from build123d import *

# Parameters (mm, degrees)
SKETCH1_W               = 70
SKETCH1_H               = 80
BOSS_EXTRUDE1_DEPTH     = 6.8
SKETCH2_W               = 54
SKETCH2_H               = 73
CUT_EXTRUDE1_DEPTH      = 107.518730747
SKETCH3_R               = 2.5
CUT_EXTRUDE2_DEPTH      = 107.518730747
LPATTERN1_COUNT         = 4
LPATTERN1_PITCH         = 16.72
MIRROR1_COPY_1_SKETCH_R = 2.5
MIRROR1_COPY_1_DEPTH    = 107.518730747
MIRROR1_COPY_2_SKETCH_R = 2.5
MIRROR1_COPY_2_DEPTH    = 107.518730747
MIRROR1_COPY_3_SKETCH_R = 2.5
MIRROR1_COPY_3_DEPTH    = 107.518730747
SKETCH5_W               = 8.11
SKETCH5_H               = 73
CUT_EXTRUDE3_DEPTH      = 2.8
SKETCH4_W               = 20
SKETCH4_H               = 8
BOSS_EXTRUDE2_DEPTH     = 6.8
SKETCH7_R               = 2.25
CUT_EXTRUDE4_DEPTH      = 6.8
FILLET1_R               = 1
FILLET2_R               = 1
FILLET3_R               = 5


with BuildPart() as part:
    # Sketch1 → Boss-Extrude1 (new body)
    with BuildSketch(Plane(origin=(0, 0, 0), x_dir=(1, 0, 0), z_dir=(0, 1, 0))):
        with Locations((35, -40)):
            Rectangle(SKETCH1_W, SKETCH1_H)
    extrude(amount=BOSS_EXTRUDE1_DEPTH)

    # Sketch2 → Cut-Extrude1 (cut, through all)
    with BuildSketch(Plane(origin=(0, 6.8, 0), x_dir=(1, 0, 0), z_dir=(0, 1, 0))):
        with Locations((35.11, -43.5)):
            Rectangle(SKETCH2_W, SKETCH2_H)
    extrude(amount=-CUT_EXTRUDE1_DEPTH, mode=Mode.SUBTRACT)

    # Sketch3 → Cut-Extrude2 (cut, through all)
    with BuildSketch(Plane(origin=(0, 6.8, 0), x_dir=(1, 0, 0), z_dir=(0, 1, 0))):
        with Locations(Location((4.055, -75.3, 0), (0, 0, 270))):
            Circle(SKETCH3_R)
    cut_extrude2 = extrude(amount=-CUT_EXTRUDE2_DEPTH, mode=Mode.SUBTRACT)

    # LPattern1: Cut-Extrude2 ×4
    with Locations(*[(0, 0, -i * LPATTERN1_PITCH) for i in range(1, LPATTERN1_COUNT)]):
        add(cut_extrude2, mode=Mode.SUBTRACT)

    # Mirror1: Cut-Extrude2 across plane
    add(cut_extrude2.mirror(Plane(origin=(35, 0, 0), x_dir=(0, 0, 1), z_dir=(1, 0, 0))), mode=Mode.SUBTRACT)

    # Mirror1 copy 1 sketch → Mirror1 copy 1 (cut, through all)
    with BuildSketch(Plane(origin=(70, 6.8, -16.72), x_dir=(-1, 0, 0), z_dir=(0, 1, 0))):
        with Locations((4.055, 75.3)):
            Circle(MIRROR1_COPY_1_SKETCH_R)
    extrude(amount=-MIRROR1_COPY_1_DEPTH, mode=Mode.SUBTRACT)

    # Mirror1 copy 2 sketch → Mirror1 copy 2 (cut, through all)
    with BuildSketch(Plane(origin=(70, 6.8, -33.44), x_dir=(-1, 0, 0), z_dir=(0, 1, 0))):
        with Locations((4.055, 75.3)):
            Circle(MIRROR1_COPY_2_SKETCH_R)
    extrude(amount=-MIRROR1_COPY_2_DEPTH, mode=Mode.SUBTRACT)

    # Mirror1 copy 3 sketch → Mirror1 copy 3 (cut, through all)
    with BuildSketch(Plane(origin=(70, 6.8, -50.16), x_dir=(-1, 0, 0), z_dir=(0, 1, 0))):
        with Locations((4.055, 75.3)):
            Circle(MIRROR1_COPY_3_SKETCH_R)
    extrude(amount=-MIRROR1_COPY_3_DEPTH, mode=Mode.SUBTRACT)

    # Sketch5 → Cut-Extrude3 (cut)
    with BuildSketch(Plane(origin=(0, 6.8, 0), x_dir=(1, 0, 0), z_dir=(0, 1, 0))):
        with Locations((4.055, -43.5)):
            Rectangle(SKETCH5_W, SKETCH5_H)
    cut_extrude3 = extrude(amount=-CUT_EXTRUDE3_DEPTH, mode=Mode.SUBTRACT)

    # Mirror2: Cut-Extrude3 across plane
    add(cut_extrude3.mirror(Plane(origin=(35, 0, 0), x_dir=(0, 0, 1), z_dir=(1, 0, 0))), mode=Mode.SUBTRACT)

    # Sketch4 → Boss-Extrude2 (add)
    with BuildSketch(Plane(origin=(0, 6.8, 0), x_dir=(1, 0, 0), z_dir=(0, 1, 0))):
        with Locations((18.11, 4)):
            Rectangle(SKETCH4_W, SKETCH4_H)
    extrude(amount=-BOSS_EXTRUDE2_DEPTH)

    # Sketch7 → Cut-Extrude4 (cut)
    with BuildSketch(Plane(origin=(0, 6.8, 0), x_dir=(1, 0, 0), z_dir=(0, 1, 0))):
        with Locations(Location((12.625606255, 3.625550083, 0), (0, 0, 270))):
            Circle(SKETCH7_R)
        with Locations(Location((23.625606255, 3.625550083, 0), (0, 0, 270))):
            Circle(SKETCH7_R)
    extrude(amount=-CUT_EXTRUDE4_DEPTH, mode=Mode.SUBTRACT)

    # Fillet1
    fillet1_edges = [part.edges().sort_by_distance(p)[0] for p in [
        (8.11, 3.4, 0),
    ]]
    fillet(fillet1_edges, radius=FILLET1_R)

    # Fillet2
    fillet2_edges = [part.edges().sort_by_distance(p)[0] for p in [
        (8.11, 3.4, -8),
        (28.11, 3.4, -8),
        (28.11, 3.4, 0),
    ]]
    fillet(fillet2_edges, radius=FILLET2_R)

    # Fillet3
    fillet3_edges = [part.edges().sort_by_distance(p)[0] for p in [
        (0, 3.4, 0),
        (70, 3.4, 0),
    ]]
    fillet(fillet3_edges, radius=FILLET3_R)


solid = part.part
Geometry: final body of the model. Coordinates: model frame, mm. A direction names the side the tool comes from. Give positions to 0.01 mm unless a question says otherwise; leave off trailing zeros. Loops run counter-clockwise (first coordinate to the right, second up) from the corner with the lowest first, then second, coordinate; pieces in that order, holes last. Notation, with made-up numbers: M 10,2 L 55,2 A27 ccw 55,28 Z; hole C 47,26.25 d10. An arc over 180 degrees is marked long. Put each result on its own line as item: value.
1) Cut plane A-A, the plane z = 75.3. Return the cut outline in (x, y) (3 decimals), plus the area to 3 significant figures.
Computed values:
outline: M 0,0 L 1.555,0 L 1.555,4 L 0,4 Z; M 6.555,0 L 8.11,0 L 8.11,4 L 6.555,4 Z; M 62.11,0 L 63.445,0 L 63.445,4 L 62.11,4 Z; M 68.445,0 L 70,0 L 70,4 L 68.445,4 Z
area: 24.0 mm^2
2) Cut plane D-D, the plane z = 2. Return the cut outline in (x, y), plus the area to 3 significant figures.
Computed values:
outline: M 1,0 L 69,0 L 69,6.8 L 1,6.8 Z
area: 462 mm^2
3) First-contact query: P1, Ø2, axis at y = 2, z = 62, coming from the -X side; P2, Ø4, axis at x = 65, z = 48, coming from the +Y side. Flat tips, straight axial feed; report the tip coordinate or a pass-through.
Computed values:
P1: stops at x = 0
P2: stops at y = 4
4) Mould query, pull axis Z, two halves, no side actions, for faces 4 (the cylindrical face through (4.806, 2.028, 44.245)), 5 (the flat face through (8.11, 3, -4)), 6 (the flat face through (6, 3, 0)). Classes: released by +Z, released by -Z, zero draft, split by the parting line, or undercut.
Computed values:
face 4: undercut
face 5: zero draft
face 6: released by -Z
5) Reachability of faces 1 (the flat face through (4, 2, 80)), 2 (the flat face through (8.11, 2, 44)), 3 (the flat face through (69, 4, 43)) from +Z, -Z, +X, -X, +Y, -Y: full face, straight path, thin tool, end or side. Return the list, or none.
Computed values:
face 1: +Z, +X, -X, +Y, -Y
face 2: +Z, +Y, -Y
face 3: +Z, +X, -X, +Y
6) Cut plane B-B, the plane z = 45.5. Return the cut outline in (x, y).
Computed values:
outline: M 0,0 L 8.11,0 L 8.11,4 L 0,4 Z; M 62.11,0 L 70,0 L 70,4 L 62.11,4 Z
7) Cut plane C-C, the plane y = 1.25. Give the number of separate pieces and of enclosed holes in the cut face, plus the area to 3 significant figures.
Computed values:
separate pieces: 1
enclosed holes: 10
area: 1,620 mm^2
8) Material intervals for L1, parallel to X at y = 3.05, z = 75.3 (3 decimals); L2, parallel to X at y = 1.5, z = 23.5; L3, parallel to X at y = 1, z = 28, sorted ascending. Write a range as from..to.
Computed values:
L1: x = 0..1.555, 6.555..8.11, 62.11..63.445, 68.445..70
L2: x = 0..2.17, 5.94..8.11, 62.11..64.06, 67.83..70
L3: x = 0..8.11, 62.11..70
